from build123d import *

# Parameters (mm, degrees)
F0_W           = 1966.9125
F0_H           = 2108.2
F1_DEPTH       = 101.6
F2_W           = 19.05
F2_H           = 50.8
F3_DEPTH       = 2108.201
F6_D           = 9.525
F6_CSINK_D     = 19.8374
F6_CSINK_ANGLE = 82


# Not quite as in the source:
# - a feature names something its author has since deleted; it is built from what else it names


with BuildPart() as f1:
    # F0 (on Front) → F1 (new body)
    with BuildSketch(Plane.XZ):
        with Locations((983.45625, 1054.1)):
            Rectangle(F0_W, F0_H)
    extrude(amount=F1_DEPTH)

    # F2 (on face) → F3 (cut, through all)
    with BuildSketch(Plane.XY.offset(2108.2)):
        with Locations((1957.3875, -25.4)):
            Rectangle(F2_W, F2_H)
    extrude(amount=-F3_DEPTH, mode=Mode.SUBTRACT)

    # F6 (through all)
    with Locations(Plane(origin=(0, 0, 0), x_dir=(-1, 0, 0), z_dir=(0, 1, 0))):
        with Locations((-1640.284375, 1854.2), (-1310.084375, 1854.2), (-656.828125, 1854.2), (-326.628125, 1854.2)):
            CounterSinkHole(F6_D / 2, F6_CSINK_D / 2, counter_sink_angle=F6_CSINK_ANGLE)


solid = f1.part
Build history of the part. All positions in model axes, mm. A direction names the side the tool comes from. Give positions to 0.01 mm unless a question says otherwise; leave off trailing zeros. Answer in a Markdown table with one row per item.
Item 1: Flat gauge pins, fed straight in: P1, Ø2, axis at x = 1068, z = 1098, coming from the +Y side; P2, Ø15, axis at x = 1640.28, z = 1854.2, coming from the +Y side. Where does each tip first touch, or does it go through?
Findings below:
| item | result |
|---|---|
| P1 | stops at y = 0 |
| P2 | stops at y = -2.78 |
Item 2: Tool access for faces 1 (the flat face through (970, -50, 0)), 2 (the flat face through (1947.862, -26, 1069)): list every direction of +Z, -Z, +X, -X, +Y, -Y with a clear straight run to the whole face (end or side of a thin tool).
Findings below:
| item | result |
|---|---|
| face 1 | -Z, +X, -X, +Y, -Y |
| face 2 | +Z, -Z, +X, +Y |
Item 3: Probe line 1 along X through (y, z) = (-51, 1854.2); line 2 along X through (y, z) = (-49, 1854.2); line 3 along Z through (x, y) = (1640.5, -9.5). List the from-to ranges inside material, lowest first. Write a range as [from, to].
Findings below:
| item | result |
|---|---|
| line 1 | x = [0, 321.87], [331.39, 652.07], [661.59, 1305.32], [1314.85, 1635.52], [1645.05, 1966.91] |
| line 2 | x = [0, 321.87], [331.39, 652.07], [661.59, 1305.32], [1314.85, 1635.52], [1645.05, 1947.86] |
| line 3 | z = [0, 1849.44], [1858.96, 2108.2] |
